The listing builds one solid part. Answer for the finished solid, in the listing's coordinates (mm). Face numbers are marked on the shaded views. Round coordinates to 2 decimals unless told otherwise and drop trailing zeros. Loops run counter-clockwise (first coordinate to the right, second up) from the corner with the lowest first, then second, coordinate; pieces in that order, holes last. Notation, with made-up numbers: (10.5, 86) -> (44.5, 86) arc R17 cw to (44.5, 116) -> close; hole circle Ø7 at (-17.5, 62.5). An arc over 180 degrees is marked (long way). One line per question, with ' | ' between items.
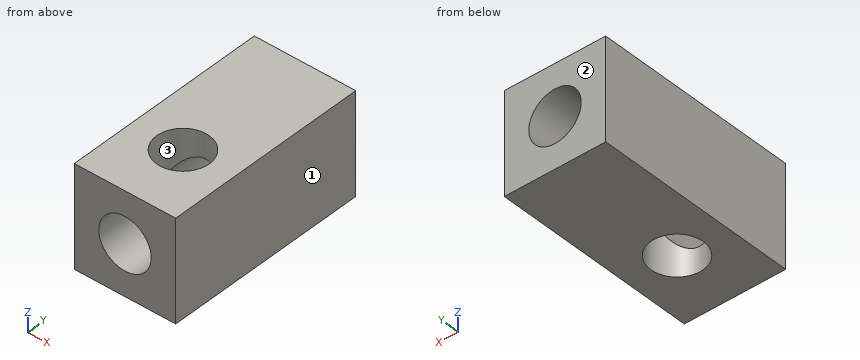
Autodesk Inventor part; units mm, degrees
ref_plane "YZ Plane" through (0, 0, 0) normal (1, 0, 0) x (0, 1, 0)
ref_plane "XZ Plane" through (0, 0, 0) normal (0, 1, 0) x (-1, 0, 0)
ref_plane "XY Plane" through (0, 0, 0) normal (0, 0, 1) x (1, 0, 0)
sketch "Sketch1" plane through (0, 0, 0) normal (0, 1, 0) x (-1, 0, 0)
  line L0 (-2.9, 2.9) -> (2.9, 2.9)
  line L1 (2.9, 2.9) -> (2.9, -2.9)
  line L2 (2.9, -2.9) -> (-2.9, -2.9)
  line L3 (-2.9, -2.9) -> (-2.9, 2.9)
  line L4 (-2.9, 2.9) -> (2.9, -2.9) construction
  line L5 (2.9, 2.9) -> (-2.9, -2.9) construction
  point P0 (0, 0)
  point P1 (0, 0)
  dimension "d0" = 5.8
extrude "Extrusion1" add sketch "Sketch1" along normal blind 11.8
hole "Hole1" at (0, 0, 0) direction (0, 1, 0) diameter 3 end through all
thread "Thread1"
sketch "Sketch2" plane through (-2.9, 0, 2.9) normal (0, 0, 1) x (1, 0, 0)
  line L0 (5.8, 0) -> (0, 0)
  line L1 (5.8, 0) -> (5.8, 11.8)
  line L2 (0, 11.8) -> (5.8, 11.8)
  line L3 (0, 0) -> (0, 11.8)
  line L4 (2.9, 0) -> (2.9, 3.8) construction
  dimension "d12" = 3.8
hole "Hole2" at (0, 3.8, 2.9) direction (0, 0, -1) diameter 3 end through all
thread "Thread2"
equation "\"square_width\" = d0"
equation "\"height\" = d1"
equation "\"side_hole_to_side_short\" = d12"
equation "\"side_hole_to_side_long\" = height - side_hole_to_side_short"
equation "\"side_hole_to_side_intermediate\" = 0.5 * square_width"
equation "\"central_hole_to_side\" = 0.5 * square_width"
properties part number "M3_cube_standoff"
Q1. Find the intervals of material crossed by line 1 (X direction, y = 8.25, z = 0); line 2 (X direction, y = 4.25, z = 2.15), in increasing order. Write a range as from..to.
Numbers:
line 1: -2.9..-1.5, 1.5..2.9 | line 2: -2.9..-1.43, 1.43..2.9
Q2. A cutting plane is placed at D-D on x = -1.1. Give the vertices of the cut face in (y, z), plus the area to 3 significant figures.
Numbers:
outline: (0, -2.9) -> (2.78, -2.9) -> (2.78, -1.02) -> (0, -1.02) -> close; (0, 1.02) -> (2.78, 1.02) -> (2.78, 2.9) -> (0, 2.9) -> close; (4.82, -2.9) -> (11.8, -2.9) -> (11.8, -1.02) -> (4.82, -1.02) -> close; (4.82, 1.02) -> (11.8, 1.02) -> (11.8, 2.9) -> (4.82, 2.9) -> close | area: 36.7 mm^2
Q3. For a pull along Y with two mould halves and no side action, classify the marked faces 1, 2 and 3 as pulls with the +Y half, pulls with the -Y half, needs draft (parallel to the pull), parting line crosses it, or undercut.
Numbers:
face 1: needs draft | face 2: pulls with the +Y half | face 3: undercut
Q4. A cutting plane is placed at B-B on z = 2.4. Give the vertices of the cut face in (x, y), plus the area to 3 significant figures.
Numbers:
outline: (-2.9, 0) -> (2.9, 0) -> (2.9, 11.8) -> (-2.9, 11.8) -> close; hole circle Ø3 at (0, 3.8) | area: 61.4 mm^2
Q5. A cutting plane is placed at C-C on y = 6.5. Give the vertices of the cut face in (x, z), plus the area to 3 significant figures.
Numbers:
outline: (-2.9, -2.9) -> (2.9, -2.9) -> (2.9, 2.9) -> (-2.9, 2.9) -> close; hole circle Ø3 at (0, 0) | area: 26.6 mm^2
Q6. A cutting plane is placed at A-A on x = 0. Give the vertices of the cut face in (y, z).
Numbers:
outline: (0, -2.9) -> (2.3, -2.9) -> (2.3, -1.5) -> (0, -1.5) -> close; (0, 1.5) -> (2.3, 1.5) -> (2.3, 2.9) -> (0, 2.9) -> close; (5.3, -2.9) -> (11.8, -2.9) -> (11.8, -1.5) -> (5.3, -1.5) -> close; (5.3, 1.5) -> (11.8, 1.5) -> (11.8, 2.9) -> (5.3, 2.9) -> close
Q7. Given pin 1 Ø2.5 at (x, z) = (0, 0) entering from -Y, flat-ended and moving along its own axis, determine where the tip first touches the part or whether it passes through.
Numbers:
pin 1: through
